Source: CAD feature listing. Evaluate the final solid. Frame: model axes, mm. Face numbers are marked on the shaded views. A direction names the side the tool comes from. Round coordinates to 2 decimals unless told otherwise and drop trailing zeros. Loops run counter-clockwise (first coordinate to the right, second up) from the corner with the lowest first, then second, coordinate; pieces in that order, holes last. Notation, with made-up numbers: (84.25, 20) -> (113.25, 20) arc R22 ccw to (113.25, 27) -> close; hole circle Ø8 at (21, 0). An arc over 180 degrees is marked (long way). Return JSON: item names as keys, results as strings. Group by question number.
Autodesk Inventor part; units mm, degrees
ref_plane "Plano de corte transversal" through (39.7887, 0, 0) normal (0, 1, 0) x (0, 0, 1)
ref_plane "Plano de trabalho2" through (0, 0, 0) normal (-1, 0, 0) x (0, 0, 1)
ref_plane "Plano de trabalho3" through (0, 300, 0) normal (-0.0628, -0.998, 0) x (0, 0, 1)
sketch "Caminho de Esboço" plane through (0, 0, 0) normal (0, 0, 1) x (1, 0, 0)
  arc A0 (-39.7887, 0) -> (39.7887, 0) centre (0, 0) ccw
  arc A1 (39.7887, 300) -> (-39.7887, 300) centre (0, 300) ccw
  line L0 (39.7887, 300) -> (39.7887, 0)
  line L1 (-39.7887, 0) -> (-39.7887, 300)
ref_plane "Plano de corte transversal" through (39.7887, 0, 0) normal (0, 1, 0) x (0, 0, 1)
ref_plane "Plano de trabalho2" through (0, 0, 0) normal (-1, 0, 0) x (0, 0, 1)
ref_plane "Plano de trabalho3" through (0, 300, 0) normal (-0.0628, -0.998, 0) x (0, 0, 1)
sketch "Seção transversal" plane through (39.7887, 0, 0) normal (0, 1, 0) x (0, 0, 1)
  line L0 (-8, 1) -> (8, 1)
  line L1 (8, 1) -> (8, -1)
  line L2 (8, -1) -> (-8, -1)
  line L3 (-8, -1) -> (-8, 1)
  line L4 (-8, 0) -> (8, 0) construction
  point P0 (0, 0)
  point P1 (0, 0)
  dimension "d0" = 16
  dimension "d4" = 1
  dimension "d5" = 1
sweep "Correia" add profiles "Seção transversal" path "Caminho de Esboço"
equation "\"d0\" = da_B"
equation "\"d4\" = da_a"
equation "\"d5\" = da_a2"
equation "\"da_B\" = 16"
equation "\"da_a\" = 1"
equation "\"da_S\" = 5.3"
equation "\"da_Beta\" = 20deg"
equation "\"da_Ht\" = 2.5"
equation "\"da_H\" = 4.5"
equation "\"da_a2\" = 1"
properties part number "Correia síncrona" material "Rubber"
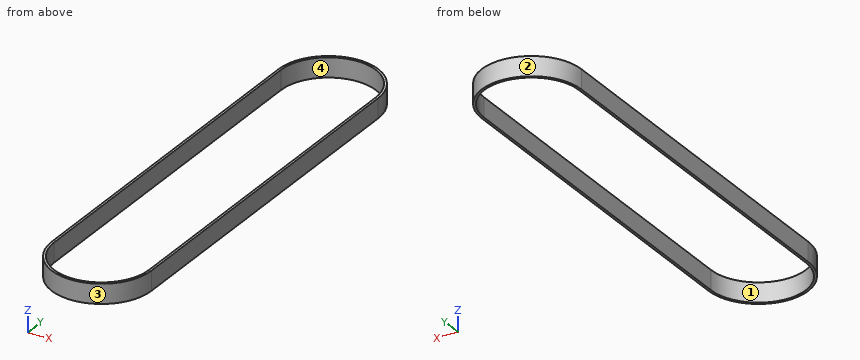
(1) Set-up query: the marked faces 3 and 4. Return all of +Z, -Z, +X, -X, +Y, -Y with unobstructed straight access to the full face (end or side cutting, diameter ignored); none if empty.
(2) Cut plane B-B (x = 0). Return loops of the section in (y, z).
(3) Ray query, line 1 (X direction, y = 215, z = -1.5); line 2 (Y direction, x = 2, z = -2.5); line 3 (Y direction, x = -1.5, z = 3). Return the intervals inside material, ascending.
(4) Mould query, pull axis X, two halves, no side actions, for the marked faces 1 and 2. Classes: released by +X, released by -X, zero draft, split by the parting line, or undercut.
(5) Pin query (flat end, axial travel): pin 1 (1.5 mm diameter, centred on x = -10, z = -2.5, fed in from +Y); pin 2 (6 mm diameter, centred on x = 32, z = 2.5, fed in from -Y); pin 3 (4 mm diameter, centred on x = -7.5, z = 0, fed in from -Y). Return the tip coordinate at first contact, or that it passes through.
(6) Cut plane C-C (y = 125). Return loops of the section in (x, z).
(7) Cut plane A-A (z = 2.5). Return loops of the section in (x, y).
Answers follow:
{
 "1": {"face 3": "+Z, -Z, -Y", "face 4": "+Z, -Z"},
 "2": {"outline": "(-40.79, -8) -> (-38.79, -8) -> (-38.79, 8) -> (-40.79, 8) -> close; (338.79, -8) -> (340.79, -8) -> (340.79, 8) -> (338.79, 8) -> close"},
 "3": {"line 1": "-40.79 to -38.79, 38.79 to 40.79", "line 2": "-40.74 to -38.74, 338.74 to 340.74", "line 3": "-40.76 to -38.76, 338.76 to 340.76"},
 "4": {"face 1": "undercut", "face 2": "split by the parting line"},
 "5": {"pin 1": "y = 339.73", "pin 2": "y = -28.68", "pin 3": "y = -40.42"},
 "6": {"outline": "(-40.79, -8) -> (-38.79, -8) -> (-38.79, 8) -> (-40.79, 8) -> close; (38.79, -8) -> (40.79, -8) -> (40.79, 8) -> (38.79, 8) -> close"},
 "7": {"outline": "(-40.79, 0) arc R40.79 ccw to (40.79, 0) -> (40.79, 300) arc R40.79 ccw to (-40.79, 300) -> close; hole (-38.79, 0) arc R38.79 ccw to (38.79, 0) -> (38.79, 300) arc R38.79 ccw to (-38.79, 300) -> close"}
}
